Here's how the part is built. I have some questions about the finished solid (model axes, mm). A direction names the side the tool comes from. Round coordinates to 2 decimals unless told otherwise and drop trailing zeros. Order: outer loops, then holes, each group sorted by start corner. A loop starts at its lowest first (then second) coordinate and runs counter-clockwise, first axis right, second up.
```python
from build123d import *

# Parameters (mm, degrees)
SKETCH1_R          = 10000
SKETCH1_R_2        = 2500
BASE_FLANGE1_DEPTH = 3400
SCALE1_SCALE       = 0.001
SKETCH2_R          = 5
CUT_EXTRUDE1_DEPTH = 216644.107193969


# Sheet-metal steps are written as plain solids
with BuildPart() as part:
    # Sketch1 → Base-Flange1 (new body)
    with BuildSketch(Plane.XY):
        Polygon((0, 0), (0, -35000), (80000, -35000), (160000, 20000), (220000, 20000), (340000, -30000), (400000, -30000), (400000, 30000), (340000, 30000), (220000, 80000), (160000, 80000), (60000, 0), align=None)
        with Locations((190000, 50000)):
            Circle(SKETCH1_R, mode=Mode.SUBTRACT)
        with Locations((280000, 25000)):
            Circle(SKETCH1_R_2, mode=Mode.SUBTRACT)
        with Locations((115000, 14570.048045386)):
            Circle(SKETCH1_R_2, mode=Mode.SUBTRACT)
    extrude(amount=-BASE_FLANGE1_DEPTH)


with BuildPart() as part_1:
    # Scale1: scaled about (215693.562550425, 18131.029763925, -1700)
    add(part.part.scale(SCALE1_SCALE).moved(Location((215477.868987875, 18112.898734161, -1698.3))))

    # Sketch2 → Cut-Extrude1 (cut, through all)
    with BuildSketch(Plane(origin=(0, 0, -1701.7), x_dir=(-1, 0, 0), z_dir=(0, 0, -1))):
        with Locations((-215486.968987875, 18090.598734161)):
            Circle(SKETCH2_R)
        with Locations((-215538.768987875, 18090.598734161)):
            Circle(SKETCH2_R)
        with Locations((-215816.968987875, 18095.598734161)):
            Circle(SKETCH2_R)
        with Locations((-215868.768987875, 18095.598734161)):
            Circle(SKETCH2_R)
    extrude(amount=-CUT_EXTRUDE1_DEPTH, mode=Mode.SUBTRACT)


solid = part_1.part
```
1. I need wall thicknesses on probe 1 along Y at (x, z) = (215527.5, -1700.45); probe 2 along X at (y, z) = (18112, -1700.7); probe 3 along X at (y, z) = (18106.5, -1701.05). Which ranges of each line are inside material? Lowest first, please.
Evaluation:
probe 1: y = 18077.9 to 18112.9
probe 2: x = 215477.87 to 215607.47, 215748.03 to 215877.87
probe 3: x = 215477.87 to 215599.47, 215761.23 to 215877.87
2. If we section it at B-B, the plane z = -1700.9: Write out the boundary of the cut face in (x, y), and give its area (3 significant figures).
Evaluation:
outline: (215477.87, 18077.9) - (215557.87, 18077.9) - (215637.87, 18132.9) - (215697.87, 18132.9) - (215817.87, 18082.9) - (215877.87, 18082.9) - (215877.87, 18142.9) - (215817.87, 18142.9) - (215697.87, 18192.9) - (215637.87, 18192.9) - (215537.87, 18112.9) - (215477.87, 18112.9) - close; hole circle Ø10 at (215486.97, 18090.6); hole circle Ø10 at (215538.77, 18090.6); hole circle Ø5 at (215592.87, 18127.47); hole circle Ø20 at (215667.87, 18162.9); hole circle Ø5 at (215757.87, 18137.9); hole circle Ø10 at (215816.97, 18095.6); hole circle Ø10 at (215868.77, 18095.6)
area: 21,100 mm2
3. If we section it at C-C, the plane x = 215554.5: Write out the boundary of the cut face in (y, z).
Evaluation:
outline: (18077.9, -1701.7) - (18126.2, -1701.7) - (18126.2, -1698.3) - (18077.9, -1698.3) - close
4. I'm going to push flat-ended pins straight in: P1, Ø1.7, axis at x = 215843, z = -1700.5, coming from the +Y side; P2, Ø1.7, axis at x = 215844.5, z = -1699.5, coming from the -Y side. Where does each tip first touch, or does it pass through?
Evaluation:
P1: stops at y = 18142.9
P2: stops at y = 18082.9
5. If we section it at A-A, the plane x = 215665: Write out the boundary of the cut face in (y, z), and give its area (3 significant figures).
Evaluation:
outline: (18132.9, -1701.7) - (18153.32, -1701.7) - (18153.32, -1698.3) - (18132.9, -1698.3) - close; (18172.48, -1701.7) - (18192.9, -1701.7) - (18192.9, -1698.3) - (18172.48, -1698.3) - close
area: 139 mm2
6. If we mould it in two halves opening along Y, with no side actions, what happens to faces 1 (the cylindrical face through (215659.933, 18156.814, -1699.976)), 2 (the flat face through (215757.03, 18108.25, -1699.98)), 3 (the flat face through (215758.71, 18167.55, -1699.98)), 4 (the flat face through (215675, 18136, -1701.7))? For each: released by +Y, released by -Y, zero draft, split by the parting line, or undercut.
Evaluation:
face 1: undercut
face 2: released by -Y
face 3: released by +Y
face 4: zero draft
7. On a 3-axis mill with a long thin cutter (end or side, diameter ignored), from which of +Z, -Z, +X, -X, +Y, -Y can I reach the whole of each face in a straight line? I mean faces 5 (the cylindrical face through (215821.964, 18095.819, -1700.024)), 6 (the flat face through (215597.309, 18105.014, -1699.976)). Say none if no direction works.
Evaluation:
face 5: +Z, -Z
face 6: +Z, -Z, -Y
